from build123d import *

# Parameters (mm, degrees)
SKETCH_1_W          = 10
SKETCH_1_H          = 25
EXTRUDE_1_DEPTH     = 0.8
SKETCH_2_R          = 2
SKETCH_2_R_2        = 1.5
EXTRUDE_2_DEPTH     = 7
SKETCH_3_R          = 1.5
CUT_EXTRUDE_1_DEPTH = 0.8


with BuildPart() as part:
    # 草图1 → 凸台-拉伸1 (new body)
    with BuildSketch(Plane.XY):
        Rectangle(SKETCH_1_W, SKETCH_1_H)
    extrude(amount=EXTRUDE_1_DEPTH)

    # 草图2 → 凸台-拉伸2 (add)
    with BuildSketch(Plane.XZ.offset(12.5)):
        with Locations((6.959591794, 0.4)):
            Circle(SKETCH_2_R)
        with Locations(Location((6.959591794, 0.4, 0), (0, 0, 270))):
            Circle(SKETCH_2_R_2, mode=Mode.SUBTRACT)
    extrude_2 = extrude(amount=-EXTRUDE_2_DEPTH)

    # 镜向1: 凸台-拉伸2 across plane
    add(extrude_2.mirror(Plane.ZX))

    # 草图3 → 切除-拉伸1 (cut)
    with BuildSketch(Plane.XY.offset(0.8)):
        with Locations((-1.020204103, 8)):
            Circle(SKETCH_3_R)
        with Locations((-1.020204103, -8)):
            Circle(SKETCH_3_R)
    extrude(amount=-CUT_EXTRUDE_1_DEPTH, mode=Mode.SUBTRACT)


solid = part.part
For this review, take the finished solid that the model builds, in its own axes (mm). A direction names the side the tool comes from. Coordinates: 2 decimals unless noted, no trailing zeros. Order: outer loops, then holes, each group sorted by start corner. A loop starts at its lowest first (then second) coordinate and runs counter-clockwise, first axis right, second up. Notation, with made-up numbers: (49.25, 19.25) - (86.25, 19.25) arc R6 ccw to (86.25, 29.25) - close; hole circle Ø4 at (41, 66). An arc over 180 degrees is marked (long way). Answer as CSV lines item,"result". Start each with the question number.
1) To check wall thickness, follow line 1 along Y through (x, z) = (5.25, 0.95); line 2 along X through (y, z) = (-8.5, 0.4); line 3 along Z through (x, y) = (-4, -6.25). State the ranges of each line that lie inside material, in increasing order. Write a range as [from, to].
2) Machinability: for faces 4 (the flat face through (0, 0, 0.8)), 5 (the flat face through (0, 0, 0)), 6 (the flat face through (3, 12.5, 0.4)), which of the approach directions +Z, -Z, +X, -X, +Y, -Y give a long, thin tool a straight path to every point of the face, cutting with its end or side? Answer none if there is none.
3) Add section D-D (x = -2). State the section outline as (y, z) points, then the cut area to 3 significant figures.
4) Insertion check: P1, Ø0.9, axis at y = -2, z = 0.5, coming from the +X side; P2, Ø1.8, axis at x = 6.96, z = 0.4, coming from the -Y side; P3, Ø3, axis at x = 1.5, y = -3.5, coming from the +Z side; P4, Ø1.5, axis at x = 4, y = 7.5, coming from the -Z side. Each pin has a flat end and moves straight along its axis. Give the tip position at first contact, or say it passes through.
5) Add section C-C (z = -0.7). State the section outline as (x, y) points.
6) Add section B-B (y = 8). State the section outline as (x, z) points.
7) Add section A-A (z = 0.4). State the section outline as (x, y) points.
8) Draft analysis for pull direction X (two halves, no side actions). For faces 1 (the flat face through (8, -5.5, -1)), 2 (the cylindrical face through (8.447, -9.049, 0.595)), 3 (the cylindrical face through (8.958, 9.049, 0.318)), state which applies: +X half, -X half, draft (parallel to the pull), parting line (faces both ways), or undercut.
Result:
1,line 1,"[-12.5, -5.5], [5.5, 12.5]"
1,line 2,"[-5, -2.43], [0.39, 5.46], [8.46, 8.96]"
1,line 3,"[0, 0.8]"
2,face 4,"+Z, -X, +Y, -Y"
2,face 5,"-Z, -X, +Y, -Y"
2,face 6,"+Z, -Z, +X, -X, +Y"
3,outline,"(-12.5, 0) - (-9.14, 0) - (-9.14, 0.8) - (-12.5, 0.8) - close; (-6.86, 0) - (6.86, 0) - (6.86, 0.8) - (-6.86, 0.8) - close; (9.14, 0) - (12.5, 0) - (12.5, 0.8) - (9.14, 0.8) - close"
3,area,"16.4 mm^2"
4,P1,"x = 5"
4,P2,"through"
4,P3,"z = 0.8"
4,P4,"z = 0"
5,outline,"(5.29, -12.5) - (5.94, -12.5) - (5.94, -5.5) - (5.29, -5.5) - close; (5.29, 5.5) - (5.94, 5.5) - (5.94, 12.5) - (5.29, 12.5) - close; (7.98, -12.5) - (8.63, -12.5) - (8.63, -5.5) - (7.98, -5.5) - close; (7.98, 5.5) - (8.63, 5.5) - (8.63, 12.5) - (7.98, 12.5) - close"
6,outline,"(-5, 0) - (-2.52, 0) - (-2.52, 0.8) - (-5, 0.8) - close; (0.48, 0) - (5, 0) arc R2 ccw (long way) to (5, 0.8) - (0.48, 0.8) - close; hole circle Ø3 at (6.96, 0.4)"
7,outline,"(-5, -12.5) - (5.46, -12.5) - (5.46, -5.5) - (5, -5.5) - (5, 5.5) - (5.46, 5.5) - (5.46, 12.5) - (-5, 12.5) - close; (8.46, -12.5) - (8.96, -12.5) - (8.96, -5.5) - (8.46, -5.5) - close; (8.46, 5.5) - (8.96, 5.5) - (8.96, 12.5) - (8.46, 12.5) - close; hole circle Ø3 at (-1.02, -8); hole circle Ø3 at (-1.02, 8)"
8,face 1,"draft"
8,face 2,"undercut"
8,face 3,"parting line"
